Part model, mm, in its own coordinate system. Give positions to 0.01 mm unless a question says otherwise; leave off trailing zeros. Order: outer loops, then holes, each group sorted by start corner. A loop starts at its lowest first (then second) coordinate and runs counter-clockwise, first axis right, second up. Notation, with made-up numbers: M 65.25,62 L 74.25,62 A14 cw 74.25,86 Z; hole C 15,86.5 d4. An arc over 180 degrees is marked long. Return JSON: item names as keys, results as strings.
from build123d import *

# Parameters (mm, degrees)
BOSS_EXTRUDE1_DEPTH = 2.5
SKETCH2_R           = 2.5
SKETCH2_R_2         = 11
SKETCH2_W           = 2.5
SKETCH2_H           = 29.5
SKETCH2_W_2         = 176
SKETCH2_H_2         = 128
CUT_EXTRUDE1_DEPTH  = 3


with BuildPart() as part:
    # Sketch1 → Boss-Extrude1 (new body)
    with BuildSketch(Plane(origin=(0, 0, 0), x_dir=(0, 0, -1), z_dir=(1, 0, 0))):
        Polygon((-245, -80), (-148.333333333, -80), (-148.333333333, -82.5), (-48.333333333, -82.5), (-48.333333333, -80), (48.333333333, -80), (48.333333333, -82.5), (148.333333333, -82.5), (148.333333333, -80), (245, -80), (245, 80), (148.333333333, 80), (148.333333333, 82.5), (48.333333333, 82.5), (48.333333333, 80), (-48.333333333, 80), (-48.333333333, 82.5), (-148.333333333, 82.5), (-148.333333333, 80), (-245, 80), align=None)
    extrude(amount=BOSS_EXTRUDE1_DEPTH)

    # Sketch2 → Cut-Extrude1 (cut)
    with BuildSketch(Plane(origin=(2.5, 0, 0), x_dir=(0, 0, -1), z_dir=(1, 0, 0))):
        with Locations((-128.333333333, 61)):
            Circle(SKETCH2_R)
        with Locations((128.333333333, 61)):
            Circle(SKETCH2_R)
        with Locations((128.333333333, -61)):
            Circle(SKETCH2_R)
        with Locations((-128.333333333, -61)):
            Circle(SKETCH2_R)
        with Locations((-223.5, 32.5)):
            Circle(SKETCH2_R)
        with Locations((-223.5, -32.5)):
            Circle(SKETCH2_R)
        with Locations((223.5, 32.5)):
            Circle(SKETCH2_R)
        with Locations((223.5, -32.5)):
            Circle(SKETCH2_R)
        with Locations((-180, 35)):
            Circle(SKETCH2_R_2)
        with Locations((-180, 0)):
            Circle(SKETCH2_R_2)
        with Locations((-180, -35)):
            Circle(SKETCH2_R_2)
        with Locations((180, 17.5)):
            Circle(SKETCH2_R_2)
        with Locations((180, 52.5)):
            Circle(SKETCH2_R_2)
        with Locations((180, -17.5)):
            Circle(SKETCH2_R_2)
        with Locations((180, -52.5)):
            Circle(SKETCH2_R_2)
        with Locations((-243.75, 32.5)):
            Rectangle(SKETCH2_W, SKETCH2_H)
        with Locations((-243.75, -32.5)):
            Rectangle(SKETCH2_W, SKETCH2_H)
        with Locations((243.75, -32.5)):
            Rectangle(SKETCH2_W, SKETCH2_H)
        with Locations((243.75, 32.5)):
            Rectangle(SKETCH2_W, SKETCH2_H)
        Rectangle(SKETCH2_W_2, SKETCH2_H_2)
    extrude(amount=-CUT_EXTRUDE1_DEPTH, mode=Mode.SUBTRACT)


solid = part.part
Q1. Band-saw the part on B-B (y = 0). Give the cut face in (x, z), then the cut area to 3 significant figures.
Established:
{"outline": "M 0,-245 L 2.5,-245 L 2.5,-88 L 0,-88 Z; M 0,88 L 2.5,88 L 2.5,169 L 0,169 Z; M 0,191 L 2.5,191 L 2.5,245 L 0,245 Z", "area": "730 mm²"}
Q2. Probe line 1 along Y through (x, z) = (1.6, 180); line 2 along Y through (x, z) = (0.9, -180); line 3 along Z through (x, y) = (0.3, 1). List the from-to ranges inside material, lowest first.
Established:
{"line 1": "y = -80 to -46, -24 to -11, 11 to 24, 46 to 80", "line 2": "y = -80 to -63.5, -41.5 to -28.5, -6.5 to 6.5, 28.5 to 41.5, 63.5 to 80", "line 3": "z = -245 to -88, 88 to 169.05, 190.95 to 245"}
Q3. Pin check, flat tips, straight feed: pin 1 (1.2 mm diameter, centred on x = 0.5, y = 33.5, fed in from -Z); pin 2 (1.2 mm diameter, centred on x = 1.5, z = 243.5, fed in from +Y). Stop position of each tip, or through.
Established:
{"pin 1": "stops at z = -242.5", "pin 2": "stops at y = 80"}
Q4. Two-plate mould, pull along Y, no slides. Class faces 1 (the flat face through (2.5, 74, 3)), 2 (the cylindrical face through (1.27, 17.98, -169.01)): +Y half, -Y half, draft (parallel to the pull), parting line (faces both ways), or undercut.
Established:
{"face 1": "draft", "face 2": "undercut"}
Q5. Band-saw the part on D-D (x = 1.6). Give the number of separate pieces and of enclosed holes in the cut face, then the cut area to 3 significant figures.
Established:
{"separate pieces": "1", "enclosed holes": "16", "area": "53,800 mm²"}
Q6. Band-saw the part on C-C (z = -32). Give the cut face in (x, y).
Established:
{"outline": "M 0,-80 L 2.5,-80 L 2.5,-64 L 0,-64 Z; M 0,64 L 2.5,64 L 2.5,80 L 0,80 Z"}
Q7. Band-saw the part on A-A (z = -180). Give the cut face in (x, y).
Established:
{"outline": "M 0,-80 L 2.5,-80 L 2.5,-63.5 L 0,-63.5 Z; M 0,-41.5 L 2.5,-41.5 L 2.5,-28.5 L 0,-28.5 Z; M 0,-6.5 L 2.5,-6.5 L 2.5,6.5 L 0,6.5 Z; M 0,28.5 L 2.5,28.5 L 2.5,41.5 L 0,41.5 Z; M 0,63.5 L 2.5,63.5 L 2.5,80 L 0,80 Z"}
